Source: three-view drawing plus pictorial views. Frame: mm from the lowest corner of the part. A direction names the side the tool comes from. Give positions to 0.01 mm unless a question says otherwise; leave off trailing zeros. Write each loop counter-clockwise with the first axis right and the second up, starting at its lowest first coordinate (ties: lowest second). Pieces come first, ordered by that corner, then holes.
Q1. Cut plane A-A on x = 8. Return the cut outline in (y, z) (1 decimal), plus the area to 3 significant figures.
Q2. Draft query along Z for the marked faces 1, 2, 3 and 4. Return one class per face: pulls with the +Z half, pulls with the -Z half, needs draft (parallel to the pull), parting line crosses it, or undercut.
Q3. Line query: L1, parallel to Z at x = 2.75, y = 36 (1 decimal); L2, parallel to Z at x = 1.5, y = 28 (1 decimal); L3, parallel to Y at x = 7.5, z = 33.5 (1 decimal). Output: solid intervals per line, ascending.
Q4. Cut plane B-B on z = 34.5. Return the cut outline in (x, y) (1 decimal).
Q5. Reachability of the marked faces 5 and 6 from +Z, -Z, +X, -X, +Y, -Y: full face, straight path, thin tool, end or side. Return the list, or none.
Q6. Pin query (flat end, axial travel): pin 1 (1 mm diameter, centred on x = 7, y = 41, fed in from -Z); pin 2 (6 mm diameter, centred on x = 3, y = 31.5, fed in from -Z) (1 decimal); pin 3 (16.5 mm diameter, centred on y = 36.5, z = 40, fed in from -X); pin 4 (6 mm diameter, centred on y = 34.5, z = 37, fed in from +X). Return the tip coordinate at first contact, or that it passes through.
Q7. Cut plane C-C on y = 9. Return the cut outline in (x, z) (1 decimal).
Q8. Cut plane D-D on z = 57.5. Return the cut outline in (x, y) (1 decimal).
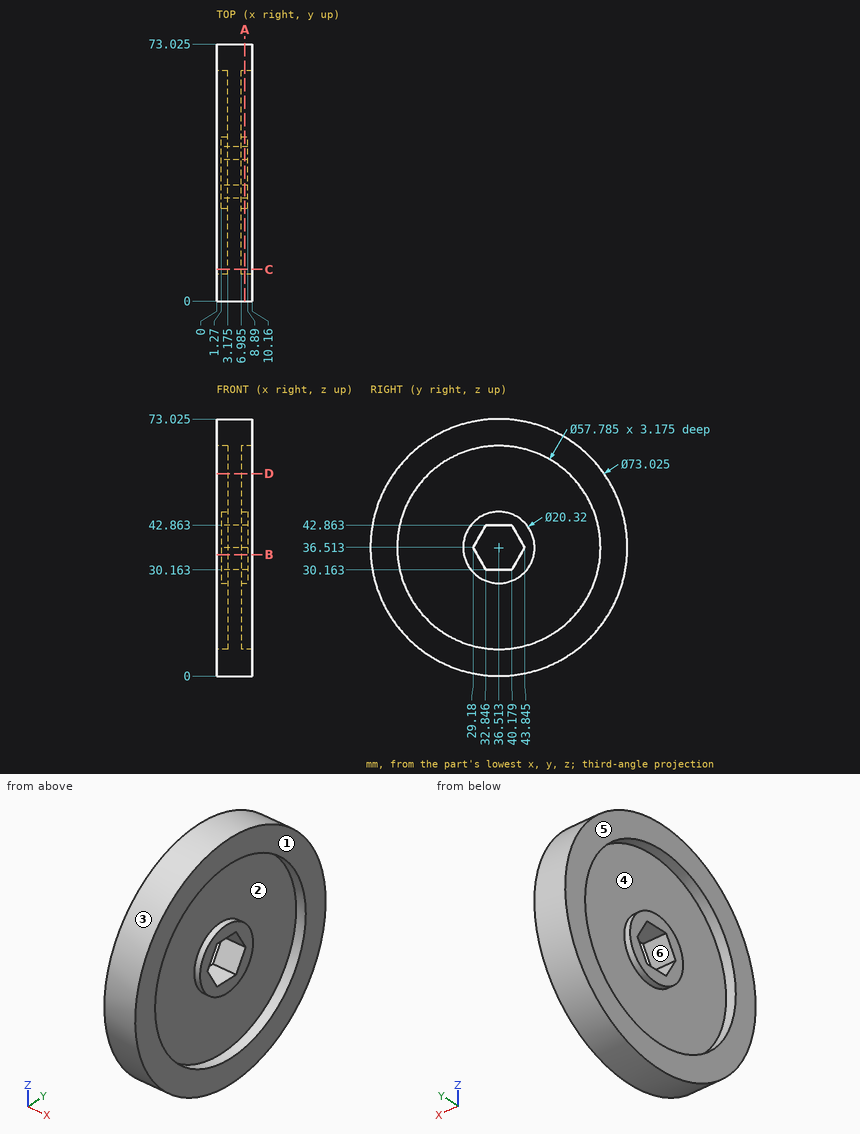
Data:
1. outline: circle Ø73 at (36.5, 36.5); circle Ø20.3 at (36.5, 36.5); hole circle Ø57.8 at (36.5, 36.5); hole (29.2, 36.5) - (32.8, 30.2) - (40.2, 30.2) - (43.8, 36.5) - (40.2, 42.9) - (32.8, 42.9) - close
1. area: 1,750 mm2
2. face 1: needs draft
2. face 2: undercut
2. face 3: parting line crosses it
2. face 4: undercut
3. L1: z = 0 to 7.6, 26.4 to 30.2, 42.9 to 46.7, 65.4 to 73
3. L2: z = 1 to 8.9, 31 to 42.1, 64.1 to 72
3. L3: y = 0.1 to 7.8, 26.8 to 30.9, 42.1 to 46.2, 65.2 to 72.9
4. outline: (0, 0.1) - (10.2, 0.1) - (10.2, 7.7) - (7, 7.7) - (7, 26.6) - (8.9, 26.6) - (8.9, 30.3) - (1.3, 30.3) - (1.3, 26.6) - (3.2, 26.6) - (3.2, 7.7) - (0, 7.7) - close; (0, 65.3) - (3.2, 65.3) - (3.2, 46.5) - (1.3, 46.5) - (1.3, 42.7) - (8.9, 42.7) - (8.9, 46.5) - (7, 46.5) - (7, 65.3) - (10.2, 65.3) - (10.2, 73) - (0, 73) - close
5. face 5: +Z, -Z, -X, +Y, -Y
5. face 6: +X, -X
6. pin 1: stops at z = 0.22
6. pin 2: stops at z = 0.1
6. pin 3: stops at x = 1.27
6. pin 4: passes through
7. outline: (0, 12.5) - (10.2, 12.5) - (10.2, 27.7) - (7, 27.7) - (7, 45.3) - (10.2, 45.3) - (10.2, 60.5) - (0, 60.5) - (0, 45.3) - (3.2, 45.3) - (3.2, 27.7) - (0, 27.7) - close
8. outline: (0, 6.6) - (10.2, 6.6) - (10.2, 16.7) - (7, 16.7) - (7, 56.4) - (10.2, 56.4) - (10.2, 66.4) - (0, 66.4) - (0, 56.4) - (3.2, 56.4) - (3.2, 16.7) - (0, 16.7) - close
